```python
from build123d import *

# Parameters (mm, degrees)
F0_W     = 67.056
F0_H     = 105.41
F1_DEPTH = 36.322
F2_R     = 5.08
F3_R     = 3.81
F4_DEPTH = 1.016


with BuildPart() as f1:
    # F0 (on Top) → F1 (new body)
    with BuildSketch(Plane.XY):
        with Locations((33.528, 52.705)):
            Rectangle(F0_W, F0_H)
    extrude(amount=F1_DEPTH)

    # F2
    f2_edges = [f1.edges().sort_by_distance(p)[0] for p in [
        (0, 0, 18.161),
        (67.056, 0, 18.161),
        (67.056, 105.41, 18.161),
        (0, 52.705, 36.322),
        (33.528, 0, 36.322),
        (67.056, 52.705, 36.322),
        (33.528, 105.41, 36.322),
        (0, 105.41, 18.161),
    ]]
    fillet(f2_edges, radius=F2_R)

    # F3 (on face) → F4 (join)
    with BuildSketch(Plane(origin=(0, 0, 0), x_dir=(1, 0, 0), z_dir=(0, 0, -1))):
        with Locations((5.08, -5.08)):
            Circle(F3_R)
        with Locations((61.976, -5.08)):
            Circle(F3_R)
        with Locations((5.08, -100.33)):
            Circle(F3_R)
        with Locations((61.976, -100.33)):
            Circle(F3_R)
    extrude(amount=F4_DEPTH)


solid = f1.part
```
For this review, take the finished solid that the model builds, in its own axes (mm). A direction names the side the tool comes from. Round coordinates to 2 decimals unless told otherwise and drop trailing zeros. Write each loop counter-clockwise with the first axis right and the second up, starting at its lowest first coordinate (ties: lowest second). Pieces come first, ordered by that corner, then holes. Notation, with made-up numbers: (45.5, -12.5) -> (53.5, -12.5) arc R4 ccw to (53.5, -7.5) -> close; hole circle Ø2 at (-5.75, 71.5). An arc over 180 degrees is marked (long way). One line per question, with ' | ' between items. Start each with the question number.
1) For pin 1 Ø20 at (x, y) = (28, 43) entering from -Z, flat-tipped, find the tip position at first contact; note if it passes through.
2) Mouldability with a two-part tool opening along Y and no side actions: class faces 1 (the cylindrical face through (1.449, 1.528, 15.84)), 2 (the cylindrical face through (33.926, 103.961, 34.794)), 3 (the cylindrical face through (58.17, 100.16, -0.5)), 4 (the flat face through (5, 100, -1.016)) as +Y half, -Y half, draft (parallel to the pull), parting line (faces both ways), or undercut.
3) Add section A-A (y = 15). Write out the cut boundary in (x, z), and give its area (3 significant figures).
4) Machinability: for faces 5 (the cylindrical face through (65.6, 53.4, 34.8)), 6 (the cylindrical face through (58.17, 4.91, -0.5)), which of the approach directions +Z, -Z, +X, -X, +Y, -Y give a long, thin tool a straight path to every point of the face, cutting with its end or side? Answer none if there is none.
5) Wall thickness on line 1 along Z through (x, y) = (52.5, 65); line 2 along X through (y, z) = (93, 31.5); line 3 along Z through (x, y) = (62, 100.5): over which ranges is each line inside the solid? List them lowest first.
6) Add section C-C (z = 33). Write out the cut boundary in (x, y), and give its area (3 significant figures).
7) Add section B-B (x = 46). Write out the cut boundary in (y, z), and give its area (3 significant figures).
Reported:
1) pin 1: stops at z = 0
2) face 1: -Y half | face 2: +Y half | face 3: undercut | face 4: draft
3) outline: (0, 0) -> (67.06, 0) -> (67.06, 31.24) arc R5.08 ccw to (61.98, 36.32) -> (5.08, 36.32) arc R5.08 ccw to (0, 31.24) -> close | area: 2,420 mm²
4) face 5: +Z, +X, +Y, -Y | face 6: -Z
5) line 1: z = 0 to 36.32 | line 2: x = 0.01 to 67.05 | line 3: z = -1.02 to 36.32
6) outline: (0.31, 5.08) arc R4.77 ccw to (5.08, 0.31) -> (61.98, 0.31) arc R4.77 ccw to (66.74, 5.08) -> (66.74, 100.33) arc R4.77 ccw to (61.98, 105.1) -> (5.08, 105.1) arc R4.77 ccw to (0.31, 100.33) -> close | area: 6,940 mm²
7) outline: (0, 0) -> (105.41, 0) -> (105.41, 31.24) arc R5.08 ccw to (100.33, 36.32) -> (5.08, 36.32) arc R5.08 ccw to (0, 31.24) -> close | area: 3,820 mm²
